from build123d import *

# Parameters (mm, degrees)
SKETCH_1_R             = 1.6
EXTRUDE_1_DEPTH        = 18
SKETCH_3_W             = 7
SKETCH_3_H             = 11.399287815
CUT_EXTRUDE_2_DEPTH    = 21.223748416
HOLE_WIZARD_M3_1_D     = 2.5
HOLE_WIZARD_M3_1_DEPTH = 3.5
HOLE_WIZARD_M3_1_TIP   = 0.751075774
CHAMFER_1_SIZE         = 1


with BuildPart() as part:
    # 草图1 → 凸台-拉伸1 (new body)
    with BuildSketch(Plane.XY):
        with BuildLine():
            Line((-3.5, -6), (-3.5, 0))
            ThreePointArc((-3.5, 0), (0, 3.5), (3.5, 0))
            Line((3.5, 0), (3.5, -6))
            Line((3.5, -6), (-3.5, -6))
        make_face()
        Circle(SKETCH_1_R, mode=Mode.SUBTRACT)
    extrude(amount=EXTRUDE_1_DEPTH)

    # 草图3 → 切除-拉伸2 (cut, through all)
    with BuildSketch(Plane.ZY.offset(3.5)):
        with Locations((9, 1.199643908)):
            Rectangle(SKETCH_3_W, SKETCH_3_H)
    extrude(amount=-CUT_EXTRUDE_2_DEPTH, mode=Mode.SUBTRACT)

    # M3 螺纹孔1
    with Locations(Plane(origin=(0, -6, 0), x_dir=(-1, 0, 0), z_dir=(0, -1, 0))):
        with Locations((0, -3), (0, -15)):
            Hole(HOLE_WIZARD_M3_1_D / 2, depth=HOLE_WIZARD_M3_1_DEPTH)
            with Locations((0, 0, -(HOLE_WIZARD_M3_1_DEPTH + HOLE_WIZARD_M3_1_TIP / 2))):  # 118° drill point
                Cone(0, HOLE_WIZARD_M3_1_D / 2, HOLE_WIZARD_M3_1_TIP, mode=Mode.SUBTRACT)

    # 倒角1
    chamfer_1_edges = [part.edges().sort_by_distance(p)[0] for p in [
        (0, -4.5, 5.5),
        (0, -4.5, 12.5),
    ]]
    chamfer(chamfer_1_edges, length=CHAMFER_1_SIZE)


solid = part.part
For this review, take the finished solid that the model builds, in its own axes (mm). A direction names the side the tool comes from. Coordinates: 2 decimals unless noted, no trailing zeros. Loops run counter-clockwise (first coordinate to the right, second up) from the corner with the lowest first, then second, coordinate; pieces in that order, holes last. Notation, with made-up numbers: (-2, 36.5) -> (27, 36.5) arc R11 cw to (27, 44.5) -> close; hole circle Ø1 at (20, 26.5). An arc over 180 degrees is marked (long way). Write each question's results on one line, items separated by ' | '.
Q1. For pin 1 Ø1 at (x, z) = (-1.5, 10) entering from +Y; pin 2 Ø1.9 at (x, y) = (0, 0) entering from -Z (3 decimals), all flat-tipped, find the tip position at first contact; note any pin that passes through.
Taken from the geometry:
pin 1: y = -4.5 | pin 2: through
Q2. Add section B-B, the plane y = 0.5. State the section outline as (x, z) points.
Taken from the geometry:
outline: (-3.46, 0) -> (-1.52, 0) -> (-1.52, 5.5) -> (-3.46, 5.5) -> close; (-3.46, 12.5) -> (-1.52, 12.5) -> (-1.52, 18) -> (-3.46, 18) -> close; (1.52, 0) -> (3.46, 0) -> (3.46, 5.5) -> (1.52, 5.5) -> close; (1.52, 12.5) -> (3.46, 12.5) -> (3.46, 18) -> (1.52, 18) -> close
Q3. Add section C-C, the plane x = 1. Count the separate pieces of the cut face and the enclosed holes in it, then the cut area to 3 significant figures.
Taken from the geometry:
separate pieces: 3 | enclosed holes: 0 | area: 76.1 mm²
Q4. To check wall thickness, follow line 1 along Z through (x, y) = (0, -3.25); line 2 along Z through (x, y) = (1, -5.5); line 3 along Z through (x, y) = (0, -4.45). State the ranges of each line that lie inside material, in increasing order. Write a range as [from, to].
Taken from the geometry:
line 1: [0, 1.75], [4.25, 5.5], [12.5, 13.75], [16.25, 18] | line 2: [0, 2.25], [3.75, 14.25], [15.75, 18] | line 3: [0, 1.75], [4.25, 6.45], [11.55, 13.75], [16.25, 18]
Q5. Machinability: for faces 1 (the cylindrical face through (-0.16, -4.23, 13.76)), 2 (the flat face through (0, -2, 12.5)), 3 (the flat face through (3.5, -5, 9)), which of the approach directions +Z, -Z, +X, -X, +Y, -Y give a long, thin tool a straight path to every point of the face, cutting with its end or side? Answer none if there is none.
Taken from the geometry:
face 1: -Y | face 2: +X, -X, +Y | face 3: +Z, -Z, +X, +Y, -Y
Q6. Mouldability with a two-part tool opening along Y and no side actions: class faces 4 (the flat face through (0, -2, 5.5)), 5 (the flat face through (0, -4, 12)), 6 (the cylindrical face through (-1.27, -0.97, 15.21)), 7 (the cylindrical face through (-1.27, -0.97, 2.71)) as +Y half, -Y half, draft (parallel to the pull), parting line (faces both ways), or undercut.
Taken from the geometry:
face 4: draft | face 5: +Y half | face 6: undercut | face 7: undercut
Q7. Add section D-D, the plane x = 2.5. State the section outline as (y, z) points.
Taken from the geometry:
outline: (-6, 0) -> (2.45, 0) -> (2.45, 5.5) -> (-3.5, 5.5) -> (-4.5, 6.5) -> (-4.5, 11.5) -> (-3.5, 12.5) -> (2.45, 12.5) -> (2.45, 18) -> (-6, 18) -> close
Q8. Add section A-A, the plane y = -2.25. State the section outline as (x, z) points.
Taken from the geometry:
outline: (-3.5, 0) -> (3.5, 0) -> (3.5, 5.5) -> (-3.5, 5.5) -> close; (-3.5, 12.5) -> (3.5, 12.5) -> (3.5, 18) -> (-3.5, 18) -> close; hole circle Ø1.67 at (0, 3); hole circle Ø1.67 at (0, 15)
